Drawing for the job (mm, zero at the part's lowest x, y, z). A direction names the side the tool comes from. Coordinates: 2 decimals unless noted, no trailing zeros. Loops run counter-clockwise (first coordinate to the right, second up) from the corner with the lowest first, then second, coordinate; pieces in that order, holes last. Notation, with made-up numbers: (12, -4.75) - (26, -4.75) arc R33 ccw to (26, 32.25) - close; hole circle Ø4 at (-9, -37). An arc over 180 degrees is marked (long way). One line per item, written item: value.
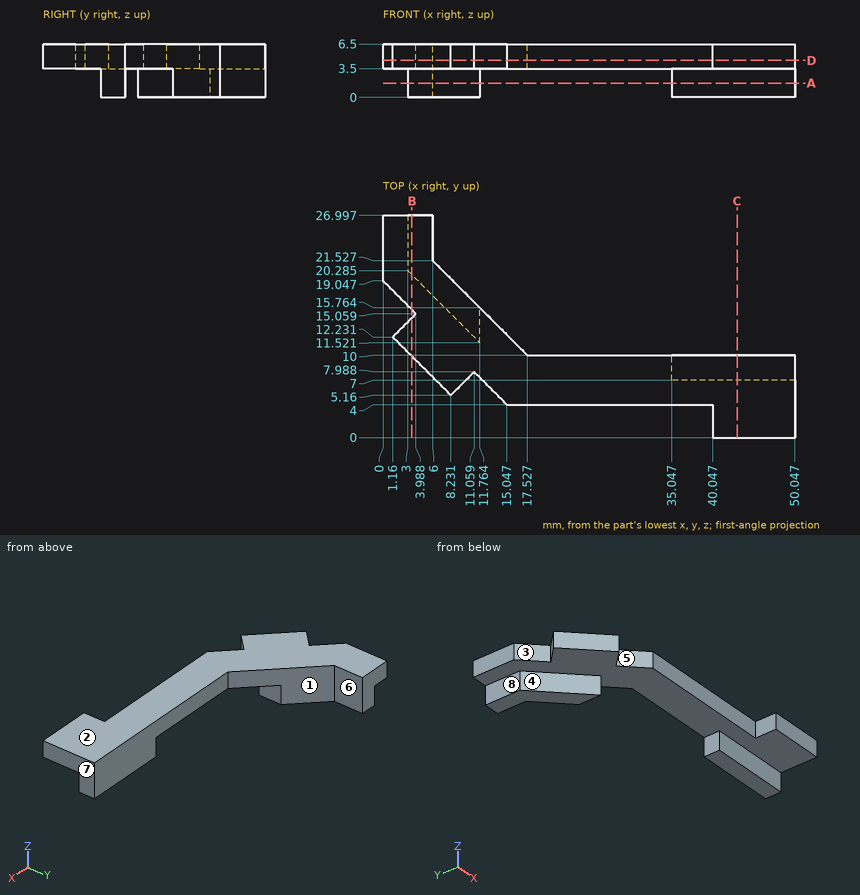
Item 1: Cut at C-C, the plane x = 43. Write the cut outline in (y, z), then the cut area to 3 significant figures.
Check result:
outline: (0, 3.5) - (7, 3.5) - (7, 0) - (10, 0) - (10, 6.5) - (0, 6.5) - close
area: 40.5 mm^2
Item 2: Cut at D-D, the plane z = 4.5. Write the cut outline in (x, y).
Check result:
outline: (0, 19.05) - (3.99, 15.06) - (1.16, 12.23) - (8.23, 5.16) - (11.06, 7.99) - (15.05, 4) - (40.05, 4) - (40.05, 0) - (50.05, 0) - (50.05, 10) - (17.53, 10) - (6, 21.53) - (6, 27) - (0, 27) - close
Item 3: Cut at A-A, the plane z = 1.75. Write the cut outline in (x, y) (1 decimal).
Check result:
outline: (3, 20.3) - (11.8, 11.5) - (11.8, 15.8) - (6, 21.5) - (6, 27) - (3, 27) - close; (35, 7) - (50, 7) - (50, 10) - (35, 10) - close
Item 4: Probe probe 1 along Y at (x, z) = (39, 4.5); probe 2 along X at (y, z) = (23.5, 2.25); probe 3 along Y at (x, z) = (45, 3.25). List the from-to ranges inside material, lowest first. Write a range as from..to.
Check result:
probe 1: y = 4..10
probe 2: x = 3..6
probe 3: y = 7..10
Item 5: Cut at B-B, the plane x = 3.5. Write the cut outline in (y, z) (1 decimal).
Check result:
outline: (9.9, 3.5) - (14.6, 3.5) - (14.6, 6.5) - (9.9, 6.5) - close; (15.5, 3.5) - (19.8, 3.5) - (19.8, 0) - (27, 0) - (27, 6.5) - (15.5, 6.5) - close
Item 6: Drop flat-ended pins along their axis: P1, Ø2.5, axis at y = 1, z = 4.5, coming from the -X side; P2, Ø2, axis at y = 14, z = 2, coming from the +X side; P3, Ø1, axis at x = 39, z = 1.5, coming from the -Y side; P4, Ø3, axis at x = 41, y = 6, coming from the -Z side. Give the stop position or say it passes through.
Check result:
P1: stops at x = 40.05
P2: stops at x = 11.76
P3: stops at y = 7
P4: stops at z = 0
Item 7: Tool access for the marked faces 5, 6, 7 and 8: list every direction of +Z, -Z, +X, -X, +Y, -Y with a clear straight run to the whole face (end or side of a thin tool).
Check result:
face 5: +Z, -Z, -Y
face 6: +Z, -Z, +X, +Y
face 7: +Z, -Z, +X, +Y, -Y
face 8: -Z, -X, +Y, -Y
Item 8: Pull direction Y, two halves, no side cores. Call the marked faces 1, 2, 3 and 4: released by +Y, released by -Y, zero draft, split by the parting line, or undercut.
Check result:
face 1: released by +Y
face 2: zero draft
face 3: undercut
face 4: released by -Y
